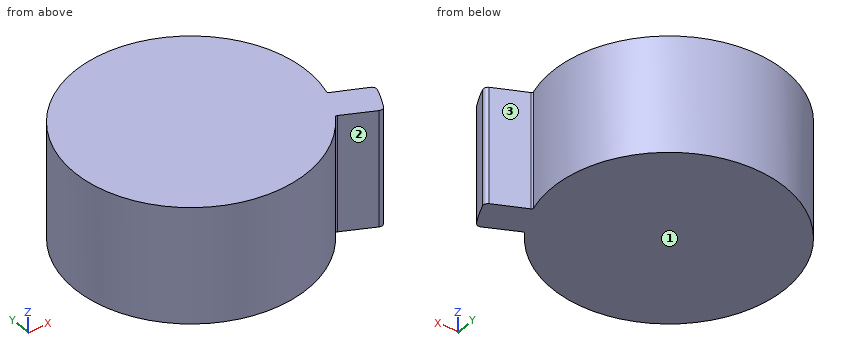
from build123d import *

# Parameters (mm, degrees)
BOSS_EXTRU_3_DEPTH = 12.5


with BuildPart() as part:
    # Esquisse1 → Boss.-Extru.3 (new body)
    with BuildSketch(Plane.XY):
        with BuildLine():
            Line((15.485185595, -5.176669047), (12.134231543, -3.650742984))
            ThreePointArc((12.134231543, -3.650742984), (12.035609724, -3.552721892), (12.024721053, -3.414100701))
            ThreePointArc((12.024721053, -3.414100701), (-11.374079439, 5.184623122), (10.464430261, -6.837082661))
            ThreePointArc((10.464430261, -6.837082661), (10.577237298, -6.754079946), (10.716830338, -6.765422852))
            Line((10.716830338, -6.765422852), (14.040747626, -8.325354826))
            ThreePointArc((14.040747626, -8.325354826), (14.40745115, -8.348324263), (14.690843755, -8.114470246))
            ThreePointArc((14.690843755, -8.114470246), (15.262737454, -6.979567539), (15.747114807, -5.80464408))
            ThreePointArc((15.747114807, -5.80464408), (15.739440197, -5.439232144), (15.485185595, -5.176669047))
        make_face()
    extrude(amount=BOSS_EXTRU_3_DEPTH)


solid = part.part
Input: part model. Units: mm. Frame: model coordinates. Face numbers are marked on the shaded views. Give positions to 0.01 mm unless a question says otherwise; leave off trailing zeros. Write each loop counter-clockwise with the first axis right and the second up, starting at its lowest first coordinate (ties: lowest second). Pieces come first, ordered by that corner, then holes. Notation, with made-up numbers: (-35.75, -9.75) -> (21.25, -9.75) arc R16 ccw to (21.25, 6.25) -> close; hole circle Ø10 at (1, -8). An arc over 180 degrees is marked (long way). Use one line per item in the form item = value. Start each with the question number.
1) Section query B-B on z = 8.5. Return the cut outline in (x, y).
2) Section query A-A on y = 0. Return the cut outline in (x, z).
3) Ray query, probe 1 along X at (y, z) = (-7.25, 11.25); probe 2 along Y at (x, z) = (-9.5, 4.5); probe 3 along Y at (x, z) = (2.5, 6). Return the intervals inside material, ascending. Write a range as from..to.
4) Pin query (flat end, axial travel): pin 1 (1.5 mm diameter, centred on y = -1.5, z = 10, fed in from -X); pin 2 (3 mm diameter, centred on y = -3, z = 5, fed in from -X); pin 3 (2 mm diameter, centred on y = 4.5, z = 1.5, fed in from +X); pin 4 (8 mm diameter, centred on x = 4, y = 6, fed in from -Z). Return the tip coordinate at first contact, or that it passes through.
5) Draft query along X for the marked faces 1, 2 and 3. Return one class per face: pulls with the +X half, pulls with the -X half, needs draft (parallel to the pull), parting line crosses it, or undercut.
6) Section query C-C on x = -3.75. Return the cut outline in (y, z).
Outcome:
q1.outline = (10.46, -6.84) arc R0.2 cw to (10.72, -6.77) -> (14.04, -8.33) arc R0.5 ccw to (14.69, -8.11) arc R16.78 ccw to (15.75, -5.8) arc R0.5 ccw to (15.49, -5.18) -> (12.13, -3.65) arc R0.2 cw to (12.02, -3.41) arc R12.5 ccw (long way) to start
q2.outline = (-12.5, 0) -> (12.5, 0) -> (12.5, 12.5) -> (-12.5, 12.5) -> close
q3.probe_1 = -10.18..10.18, 11.75..15.14
q3.probe_2 = -8.12..8.12
q3.probe_3 = -12.25..12.25
q4.pin_1 = -12.48
q4.pin_2 = -12.41
q4.pin_3 = 12
q4.pin_4 = 0
q5.face_1 = needs draft
q5.face_2 = undercut
q5.face_3 = pulls with the +X half
q6.outline = (-11.92, 0) -> (11.92, 0) -> (11.92, 12.5) -> (-11.92, 12.5) -> close
